```python
from build123d import *

# Parameters (mm, degrees)
F0_W     = 50.8
F0_H     = 25.4
F1_DEPTH = 6.35
F2_W     = 6.477
F2_H     = 6.477
F2_W_2   = 6.35
F2_H_2   = 6.35
F2_W_3   = 6.223
F2_H_3   = 6.223
F3_DEPTH = 25.4
F4_R     = 5.08


with BuildPart() as f1:
    # F0 (on Top) → F1 (new body)
    with BuildSketch(Plane.XY):
        with Locations((25.4, 12.7)):
            Rectangle(F0_W, F0_H)
    extrude(amount=F1_DEPTH)

    # F2 (on face) → F3 (cut)
    with BuildSketch(Plane.XY.offset(6.35)):
        with Locations((12.7, 12.7)):
            Rectangle(F2_W, F2_H)
        with Locations((25.4, 12.7)):
            Rectangle(F2_W_2, F2_H_2)
        with Locations((38.1, 12.7)):
            Rectangle(F2_W_3, F2_H_3)
    extrude(amount=-F3_DEPTH, mode=Mode.SUBTRACT)

    # F4
    f4_edges = [f1.edges().sort_by_distance(p)[0] for p in [
        (0, 25.4, 3.175),
        (0, 0, 3.175),
        (50.8, 25.4, 3.175),
        (50.8, 0, 3.175),
    ]]
    fillet(f4_edges, radius=F4_R)


solid = f1.part
```
Could you check a few things on this model? Use its own coordinates, in mm. A direction names the side the tool comes from. Round coordinates to 2 decimals unless told otherwise and drop trailing zeros. Order: outer loops, then holes, each group sorted by start corner. A loop starts at its lowest first (then second) coordinate and runs counter-clockwise, first axis right, second up. Notation, with made-up numbers: (-8.5, 23) -> (17.5, 23) arc R13 ccw to (17.5, 35) -> close; hole circle Ø7 at (67.25, 65.5). An arc over 180 degrees is marked (long way). One line per question, with ' | ' between items.
Q1. If we section it at B-B on z = 1.75: Write out the boundary of the cut face in (x, y) (1 decimal).
Computed values:
outline: (0, 5.1) arc R5.1 ccw to (5.1, 0) -> (45.7, 0) arc R5.1 ccw to (50.8, 5.1) -> (50.8, 20.3) arc R5.1 ccw to (45.7, 25.4) -> (5.1, 25.4) arc R5.1 ccw to (0, 20.3) -> close; hole (9.5, 9.5) -> (15.9, 9.5) -> (15.9, 15.9) -> (9.5, 15.9) -> close; hole (22.2, 9.5) -> (28.6, 9.5) -> (28.6, 15.9) -> (22.2, 15.9) -> close; hole (35, 9.6) -> (41.2, 9.6) -> (41.2, 15.8) -> (35, 15.8) -> close
Q2. If I drill on line 1 (X direction, y = 14.25, z = 3) (1 decimal); line 2 (Y direction, x = 15.5, z = 5.5); line 3 (Y direction, x = 40, z = 4.25), over which ranges is the centre line in solid material (lowest first)? Write a range as from..to.
Computed values:
line 1: 0..9.5, 15.9..22.2, 28.6..35, 41.2..50.8 | line 2: 0..9.46, 15.94..25.4 | line 3: 0..9.59, 15.81..25.4
Q3. If we section it at A-A on y = 15.25: Give the number of separate pieces and of enclosed holes in the cut face, plus the area to 3 significant figures.
Computed values:
separate pieces: 4 | enclosed holes: 0 | area: 202 mm²
Q4. If we section it at C-C on x = 14: Write out the boundary of the cut face in (y, z).
Computed values:
outline: (0, 0) -> (9.46, 0) -> (9.46, 6.35) -> (0, 6.35) -> close; (15.94, 0) -> (25.4, 0) -> (25.4, 6.35) -> (15.94, 6.35) -> close
Q5. We'd pull the mould along X, two halves only. Please class faces 3 (the face through (31, 13, 0)), 4 (the face through (28.575, 13, 3)), 5 (the face through (49.272, 1.449, 3.219)), 6 (the face through (22.225, 13, 3)): released by +X, released by -X, zero draft, split by the parting line, or undercut.
Computed values:
face 3: zero draft | face 4: undercut | face 5: released by +X | face 6: undercut
Q6. I'm going to push a flat-ended pin straight in: pin 1 (5 mm diameter, centred on x = 39, y = 22.5, fed in from -Z). Where does the tip first touch, or does it pass through?
Computed values:
pin 1: z = 0
Q7. Which directions (+Z, -Z, +X, -X, +Y, -Y) give clear straight access to the entire face, cutting with the end or side of a thin tool? Please do faces 1 (the face through (25, 15.875, 3)), 2 (the face through (1.449, 1.528, 3.219)).
Computed values:
face 1: +Z, -Z | face 2: +Z, -Z, -X, -Y
